from build123d import *

# Parameters (mm, degrees)
SKETCH1_W           = 21
SKETCH1_H           = 6
BOSS_EXTRUDE1_DEPTH = 18
BOSS_EXTRUDE2_DEPTH = 18
FILLET1_R           = 1


with BuildPart() as part:
    # Sketch1 → Boss-Extrude1 (new body)
    with BuildSketch(Plane(origin=(0, 0, 0), x_dir=(1, 0, 0), z_dir=(0, 1, 0))):
        Rectangle(SKETCH1_W, SKETCH1_H)
    extrude(amount=BOSS_EXTRUDE1_DEPTH)

    # Sketch2 → Boss-Extrude2 (add)
    with BuildSketch(Plane(origin=(0, 18, 0), x_dir=(1, 0, 0), z_dir=(0, 1, 0))):
        with BuildLine():
            Line((-10.5, 3), (-8.127429358, 3))
            ThreePointArc((-8.127429358, 3), (-25.982441938, 0.879268272), (-8.857121606, -4.6))
            Line((-8.857121606, -4.6), (-10.762377494, -3.5))
            ThreePointArc((-10.762377494, -3.5), (-23.818859397, 0.282330458), (-10.5, 3))
        make_face()
        with BuildLine():
            Line((10.762377494, -3.5), (8.857121606, -4.6))
            ThreePointArc((8.857121606, -4.6), (25.982441938, 0.879268272), (8.127429358, 3))
            Line((8.127429358, 3), (10.5, 3))
            ThreePointArc((10.5, 3), (23.818859397, 0.282330458), (10.762377494, -3.5))
        make_face()
    extrude(amount=-BOSS_EXTRUDE2_DEPTH)

    # Fillet1
    fillet1_edges = [part.edges().sort_by_distance(p)[0] for p in [
        (-10.762377494, 9, 3.5),
        (-8.857121606, 9, 4.6),
        (8.857121606, 9, 4.6),
        (10.762377494, 9, 3.5),
    ]]
    fillet(fillet1_edges, radius=FILLET1_R)


solid = part.part
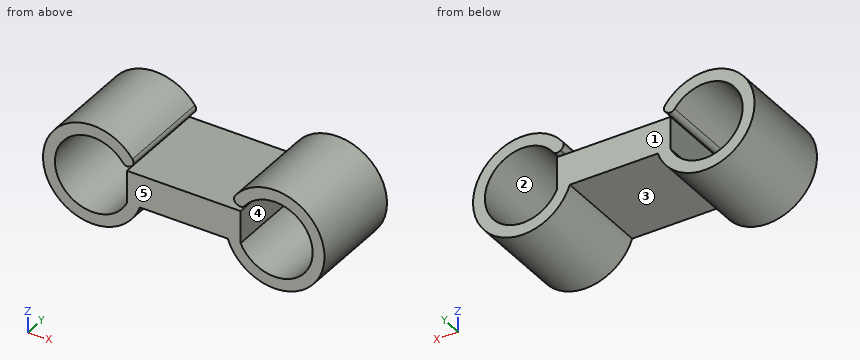
Read the model definition and answer for the solid it produces. Units are mm, in the model's axes. Face numbers are marked on the shaded views. A direction names the side the tool comes from. Round coordinates to 2 decimals unless told otherwise and drop trailing zeros. Write each loop counter-clockwise with the first axis right and the second up, starting at its lowest first coordinate (ties: lowest second). Pieces come first, ordered by that corner, then holes.
Q1. Find section C-C on z = -5.5. Determine the outline of the cut face in (x, y).
Values:
outline: (-24.2, 0) - (-21.15, 0) - (-21.15, 18) - (-24.2, 18) - close; (-12.49, 0) - (-9.45, 0) - (-9.45, 18) - (-12.49, 18) - close; (9.45, 0) - (12.49, 0) - (12.49, 18) - (9.45, 18) - close; (21.15, 0) - (24.2, 0) - (24.2, 18) - (21.15, 18) - close
Q2. Flat-ended cylindrical pins translate along their axes: P1, Ø10, axis at x = -11.5, y = 8, coming from the -Z side; P2, Ø1.5, axis at y = 15.5, z = 3.5, coming from the +X side; P3, Ø3, axis at x = 13, y = 8, coming from the +Z side. Find the tip coordinate at first contact, or state that the pin passes through.
Values:
P1: stops at z = -9.19
P2: stops at x = 25.6
P3: stops at z = 8.9
Q3. Find section B-B on x = 15.5. Determine the outline of the cut face in (y, z), and give its area (3 significant figures).
Values:
outline: (0, -9.1) - (18, -9.1) - (18, -6.87) - (0, -6.87) - close; (0, 6.87) - (18, 6.87) - (18, 9.1) - (0, 9.1) - close
area: 80.3 mm2
Q4. A tool of negligible diameter and unlimited length cuts with its end or side. For the marked faces 3, 4 and 5, from which of +Z, -Z, +X, -X, +Y, -Y can it reach the whole face along a straight path? Write none if from no direction.
Values:
face 3: -Z, +Y, -Y
face 4: +Y, -Y
face 5: +Z, -Z, +X, -X, -Y
Q5. Find section A-A on z = 0. Determine the outline of the cut face in (x, y).
Values:
outline: (-26.02, 0) - (-23.82, 0) - (-23.82, 18) - (-26.02, 18) - close; (-10.5, 0) - (10.5, 0) - (10.5, 18) - (-10.5, 18) - close; (23.82, 0) - (26.02, 0) - (26.02, 18) - (23.82, 18) - close
Q6. Find section D-D on x = -3. Determine the outline of the cut face in (y, z).
Values:
outline: (0, -3) - (18, -3) - (18, 3) - (0, 3) - close
Q7. Straight lines are drawn through the part: line 1 (X direction, y = 5.25, z = 0); line 2 (X direction, y = 11.5, z = 2); line 3 (Z direction, x = 22.5, y = 1.75). For each, find the intervals that lie inside material, in ascending order.
Values:
line 1: x = -26.02 to -23.82, -10.5 to 10.5, 23.82 to 26.02
line 2: x = -25.8 to -23.53, -10.5 to 10.5, 23.53 to 25.8
line 3: z = -7.24 to -4.1, 4.1 to 7.24
Q8. The mould has two halves that part along X. Classify the marked faces 1 and 2: released by +X, released by -X, zero draft, split by the parting line, or undercut.
Values:
face 1: zero draft
face 2: undercut
